Design review of the part built by this model. Coordinates are the model's own, in mm. Give positions to 0.01 mm unless a question says otherwise; leave off trailing zeros. Loops run counter-clockwise (first coordinate to the right, second up) from the corner with the lowest first, then second, coordinate; pieces in that order, holes last.
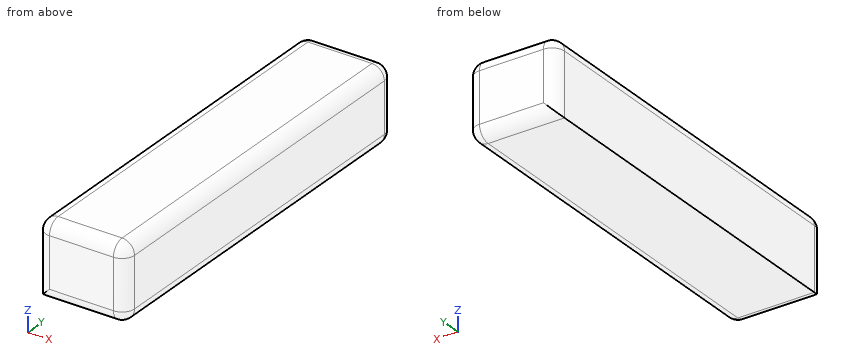
from build123d import *

# Parameters (mm, degrees)
F0_W     = 36.322
F0_H     = 157.48
F1_DEPTH = 30.734
F2_R     = 5.08


with BuildPart() as f1:
    # F0 (on Top) → F1 (new body)
    with BuildSketch(Plane.XY):
        with Locations((-35.529498, 14.489323)):
            Rectangle(F0_W, F0_H)
    extrude(amount=F1_DEPTH)

    # F2
    f2_edges = [f1.edges().sort_by_distance(p)[0] for p in [
        (-53.690498, -64.250677, 15.367),
        (-17.368498, -64.250677, 15.367),
        (-35.529498, -64.250677, 0),
        (-35.529498, -64.250677, 30.734),
        (-17.368498, 93.229323, 15.367),
        (-53.690498, 93.229323, 15.367),
        (-35.529498, 93.229323, 30.734),
        (-35.529498, 93.229323, 0),
        (-53.690498, 14.489323, 30.734),
        (-17.368498, 14.489323, 30.734),
        (-17.368498, 14.489323, 0),
    ]]
    fillet(f2_edges, radius=F2_R)


solid = f1.part
Q1. Take a section at A-A (x = -20). Give the boundary of the cut face in (y, z), plus the area to 3 significant figures.
Results:
outline: (-63.62, 5.08) arc R4.45 ccw to (-59.17, 0.63) - (88.15, 0.63) arc R4.45 ccw to (92.6, 5.08) - (92.6, 25.65) arc R4.45 ccw to (88.15, 30.1) - (-59.17, 30.1) arc R4.45 ccw to (-63.62, 25.65) - close
area: 4,590 mm2
Q2. Wall thickness on line 1 (X direction, y = 72.5, z = 26); line 2 (Y direction, x = -22, z = 17); line 3 (X direction, y = -35.5, z = 2.5): over which ranges is each line inside the solid? List them lowest first.
Results:
line 1: x = -53.68 to -17.38
line 2: y = -64.23 to 93.21
line 3: x = -53.69 to -18.07
Q3. Insertion check: pin 1 (1 mm diameter, centred on x = -22, y = -42.5, fed in from -Z); pin 2 (1 mm diameter, centred on x = -49.5, z = 8.5, fed in from -Y). Each pin has a flat end and moves straight along its axis. Give the tip position at first contact, or say it passes through.
Results:
pin 1: stops at z = 0
pin 2: stops at y = -64.24
Q4. Take a section at B-B (z = 3). Give the boundary of the cut face in (x, y), plus the area to 3 significant figures.
Results:
outline: (-53.69, -59.17) arc R5.08 ccw to (-50.69, -63.81) - (-22.45, -63.81) arc R4.63 ccw to (-17.81, -59.17) - (-17.81, 88.15) arc R4.63 ccw to (-22.45, 92.78) - (-50.69, 92.78) arc R5.08 ccw to (-53.69, 88.15) - close
area: 5,600 mm2
